```python
from build123d import *

# Parameters (mm, degrees)
SKETCH_1_R          = 14.25
EXTRUDE_1_DEPTH     = 17
SKETCH_2_R          = 10
EXTRUDE_2_DEPTH     = 30
CUT_EXTRUDE_1_DEPTH = 52.138292893
SKETCH_4_R          = 7
CUT_EXTRUDE_2_DEPTH = 52.123690078


with BuildPart() as part:
    # 草图1 → 拉伸1 (new body)
    with BuildSketch(Plane.XY):
        Circle(SKETCH_1_R)
    extrude(amount=EXTRUDE_1_DEPTH)

    # 草图2 → 拉伸2 (add)
    with BuildSketch(Plane.XY.offset(17)):
        Circle(SKETCH_2_R)
    extrude(amount=EXTRUDE_2_DEPTH)

    # 草图3 → 切除-拉伸1 (cut, through all)
    with BuildSketch(Plane(origin=(0, 0, 0), x_dir=(-1, 0, 0), z_dir=(0, 0, -1))):
        with BuildLine():
            Line((2.950875682, 10.385318132), (4.815820141, 9.6628348))
            Line((4.815820141, 9.6628348), (7.422273255, 12.164388999))
            ThreePointArc((7.422273255, 12.164388999), (5.147693743, 13.287729269), (2.709969755, 13.989945101))
            Line((2.709969755, 13.989945101), (2.950875682, 10.385318132))
        make_face()
        with BuildLine():
            Line((-1, 10.75), (1, 10.75))
            Line((1, 10.75), (2.526779539, 14.024189287))
            ThreePointArc((2.526779539, 14.024189287), (0, 14.25), (-2.526779539, 14.024189287))
            Line((-2.526779539, 14.024189287), (-1, 10.75))
        make_face()
        with BuildLine():
            Line((6.503219252, 8.618041504), (7.981237086, 7.270650216))
            Line((7.981237086, 7.270650216), (11.315347839, 8.661720572))
            ThreePointArc((11.315347839, 8.661720572), (9.600162922, 10.53087707), (7.580722617, 12.066281308))
            Line((7.580722617, 12.066281308), (6.503219252, 8.618041504))
        make_face()
        with BuildLine():
            Line((9.177267026, 5.686850616), (10.068743738, 3.896524033))
            Line((10.068743738, 3.896524033), (13.680221998, 3.989238785))
            ThreePointArc((13.680221998, 3.989238785), (12.756076902, 6.35177157), (11.427656884, 8.512999362))
            Line((11.427656884, 8.512999362), (9.177267026, 5.686850616))
        make_face()
        with BuildLine():
            Line((10.611874036, 1.987619041), (10.796410755, -0.003849312))
            Line((10.796410755, -0.003849312), (14.197506371, -1.222011804))
            ThreePointArc((14.197506371, -1.222011804), (14.189212012, 1.314824122), (13.731222765, 3.809989681))
            Line((13.731222765, 3.809989681), (10.611874036, 1.987619041))
        make_face()
        with BuildLine():
            Line((10.613288654, -1.9800515), (10.065962674, -3.903702786))
            Line((10.065962674, -3.903702786), (12.797338837, -6.268222929))
            ThreePointArc((12.797338837, -6.268222929), (13.706015415, -3.899697609), (14.180310925, -1.407580219))
            Line((14.180310925, -1.407580219), (10.613288654, -1.9800515))
        make_face()
        with BuildLine():
            Line((9.18131983, -5.680305114), (7.976050557, -7.276339568))
            Line((7.976050557, -7.276339568), (9.668819781, -10.467875813))
            ThreePointArc((9.668819781, -10.467875813), (11.371745489, -8.587543568), (12.714269518, -6.43504861))
            Line((12.714269518, -6.43504861), (9.18131983, -5.680305114))
        make_face()
        with BuildLine():
            Line((6.509362887, -8.613402046), (4.808928615, -9.666266372))
            Line((4.808928615, -9.666266372), (5.234473037, -13.253784064))
            ThreePointArc((5.234473037, -13.253784064), (7.501658321, -12.115594184), (9.531095561, -10.593428029))
            Line((9.531095561, -10.593428029), (6.509362887, -8.613402046))
        make_face()
        with BuildLine():
            Line((2.958280416, -10.383211304), (0.992334217, -10.750710339))
            Line((0.992334217, -10.750710339), (0.093181704, -14.249695336))
            ThreePointArc((0.093181704, -14.249695336), (2.618430629, -14.00736667), (5.060694335, -13.321106292))
            Line((5.060694335, -13.321106292), (2.958280416, -10.383211304))
        make_face()
        with BuildLine():
            Line((-0.992334217, -10.750710339), (-2.958280416, -10.383211304))
            Line((-2.958280416, -10.383211304), (-5.060694335, -13.321106292))
            ThreePointArc((-5.060694335, -13.321106292), (-2.618430629, -14.00736667), (-0.093181704, -14.249695336))
            Line((-0.093181704, -14.249695336), (-0.992334217, -10.750710339))
        make_face()
        with BuildLine():
            Line((-4.808928615, -9.666266372), (-6.509362887, -8.613402046))
            Line((-6.509362887, -8.613402046), (-9.531095561, -10.593428029))
            ThreePointArc((-9.531095561, -10.593428029), (-7.501658321, -12.115594184), (-5.234473037, -13.253784064))
            Line((-5.234473037, -13.253784064), (-4.808928615, -9.666266372))
        make_face()
        with BuildLine():
            Line((-7.976050557, -7.276339568), (-9.18131983, -5.680305114))
            Line((-9.18131983, -5.680305114), (-12.714269518, -6.43504861))
            ThreePointArc((-12.714269518, -6.43504861), (-11.371745489, -8.587543568), (-9.668819781, -10.467875813))
            Line((-9.668819781, -10.467875813), (-7.976050557, -7.276339568))
        make_face()
        with BuildLine():
            Line((-10.065962674, -3.903702786), (-10.613288654, -1.9800515))
            Line((-10.613288654, -1.9800515), (-14.180310925, -1.407580219))
            ThreePointArc((-14.180310925, -1.407580219), (-13.706015415, -3.899697609), (-12.797338837, -6.268222929))
            Line((-12.797338837, -6.268222929), (-10.065962674, -3.903702786))
        make_face()
        with BuildLine():
            Line((-10.796410755, -0.003849312), (-10.611874036, 1.987619041))
            Line((-10.611874036, 1.987619041), (-13.731222765, 3.809989681))
            ThreePointArc((-13.731222765, 3.809989681), (-14.189212012, 1.314824122), (-14.197506371, -1.222011804))
            Line((-14.197506371, -1.222011804), (-10.796410755, -0.003849312))
        make_face()
        with BuildLine():
            Line((-10.068743738, 3.896524033), (-9.177267026, 5.686850616))
            Line((-9.177267026, 5.686850616), (-11.427656884, 8.512999362))
            ThreePointArc((-11.427656884, 8.512999362), (-12.756076902, 6.35177157), (-13.680221998, 3.989238785))
            Line((-13.680221998, 3.989238785), (-10.068743738, 3.896524033))
        make_face()
        with BuildLine():
            Line((-7.981237086, 7.270650216), (-6.503219252, 8.618041504))
            Line((-6.503219252, 8.618041504), (-7.580722617, 12.066281308))
            ThreePointArc((-7.580722617, 12.066281308), (-9.600162922, 10.53087707), (-11.315347839, 8.661720572))
            Line((-11.315347839, 8.661720572), (-7.981237086, 7.270650216))
        make_face()
        with BuildLine():
            Line((-4.815820141, 9.6628348), (-2.950875682, 10.385318132))
            Line((-2.950875682, 10.385318132), (-2.709969755, 13.989945101))
            ThreePointArc((-2.709969755, 13.989945101), (-5.147693743, 13.287729269), (-7.422273255, 12.164388999))
            Line((-7.422273255, 12.164388999), (-4.815820141, 9.6628348))
        make_face()
    extrude(amount=-CUT_EXTRUDE_1_DEPTH, mode=Mode.SUBTRACT)

    # 草图4 → 切除-拉伸2 (cut, through all)
    with BuildSketch(Plane.XY.offset(47)):
        Circle(SKETCH_4_R)
    extrude(amount=-CUT_EXTRUDE_2_DEPTH, mode=Mode.SUBTRACT)


solid = part.part
```
Can you work these out from the model? Positions are in its coordinate system, mm. A direction names the side the tool comes from. Coordinates: 2 decimals unless noted, no trailing zeros. Write each loop counter-clockwise with the first axis right and the second up, starting at its lowest first coordinate (ties: lowest second). Pieces come first, ordered by that corner, then holes. Notation, with made-up numbers: M 24.5,-30.5 L 69.5,-30.5 A20 cw 69.5,-18.5 Z; hole C -24.75,50.25 d7. An arc over 180 degrees is marked long. Write item = value, one per line. Start each with the question number.
Q1. Thinking about a two-plate mould opening in Y: for faces 1 (the face through (-1.989, -10.564, 8.381)), 2 (the face through (2.832, 12.162, 8.381)), 3 (the face through (-8.587, -6.467, 8.381)), which applies, released by +Y, released by -Y, zero draft, split by the parting line, or undercut?
Q2. If we section it at D-D, the plane x = -12: Write out the boundary of the cut face in (y, z).
Q3. I'm going to push flat-ended pins straight in: pin 1 (8 mm diameter, centred on y = 3.5, z = 6, fed in from +X); pin 2 (0.6 mm diameter, centred on x = 0.5, z = 9, fed in from +Y); pin 3 (2 mm diameter, centred on x = 4, y = -6.5, fed in from -Z); pin 4 (5 mm diameter, centred on y = -9.5, z = 10.5, fed in from +X). Where does each tip first touch, or does it pass through?
Q4. If I drill on L1, parallel to Y at x = 0, z = 10; L2, parallel to Y at x = -12, z = 8; L3, parallel to Y at x = 0, z = 34.5, over which ranges is the centre line in solid material (lowest first)? Write a range as [from, to].
Q5. If we section it at B-B, the plane y = -12.25: Write out the boundary of the cut face in (x, z), then the cut area to 3 significant figures.
Q6. If we section it at C-C, the plane z = 18.5: Write out the boundary of the cut face in (x, y), then the cut area to 3 significant figures.
Q7. On a 3-axis mill with a long thin cutter (end or side, diameter ignored), from which of +Z, -Z, +X, -X, +Y, -Y can I reach the whole of each face in a straight line? I mean faces 4 (the face through (8.57, -6.49, 8.38)), 5 (the face through (10.3, 7.1, 8.4)), 6 (the face through (-1.75, 12.36, 8.38)), 7 (the face through (-10.343, -2.928, 8.381)). Say none if no direction works.
Q8. If we section it at A-A, the plane x = 2: Write out the boundary of the cut face in (y, z).
Check sheet entries:
q1.face_1 = released by -Y
q1.face_2 = released by +Y
q1.face_3 = undercut
q2.outline = M -6.28,0 L -5.58,0 L -5.58,17 L -6.28,17 Z; M -1.76,0 L -0.43,0 L -0.43,17 L -1.76,17 Z; M 2.8,0 L 3.95,0 L 3.95,17 L 2.8,17 Z
q3.pin_1 = 13.73
q3.pin_2 = 10.75
q3.pin_3 = 0
q3.pin_4 = 9.67
q4.L1 = [-14.25, -7], [7, 10.75]
q4.L2 = [-6.28, -5.58], [-1.76, -0.43], [2.8, 3.95]
q4.L3 = [-10, -7], [7, 10]
q5.outline = M -5.12,0 L -4.29,0 L -4.29,17 L -5.12,17 Z; M -0.61,0 L 0.61,0 L 0.61,17 L -0.61,17 Z; M 4.29,0 L 5.12,0 L 5.12,17 L 4.29,17 Z
q5.area = 48.6 mm²
q6.outline = C 0,0 d20; hole C 0,0 d14
q6.area = 160 mm²
q7.face_4 = +Z, -Z
q7.face_5 = +Z, -Z, +X
q7.face_6 = +Z, -Z, +Y
q7.face_7 = +Z, -Z, -X
q8.outline = M -10.56,0 L -6.71,0 L -6.71,47 L -9.8,47 L -9.8,17 L -10.56,17 Z; M 6.71,0 L 12.89,0 L 12.89,17 L 9.8,17 L 9.8,47 L 6.71,47 Z
